Check sheet for the modelled part. Datum: model origin and axes. Units: mm. A direction names the side the tool comes from. Round coordinates to 2 decimals unless told otherwise and drop trailing zeros. Loops run counter-clockwise (first coordinate to the right, second up) from the corner with the lowest first, then second, coordinate; pieces in that order, holes last. Notation, with made-up numbers: (44, 53.5) - (76, 53.5) arc R22 ccw to (76, 81.5) - close; hole circle Ø5 at (13, 69). An arc over 180 degrees is marked (long way). Answer in a Markdown table with one row per item. Add a question column.
(1) Mould release check, pull along Z, two halves, no side actions. Record for faces 1 (the flat face through (2, -129, 637.838)), 2 (the flat face through (2, -905, 0)), 3 (the cylindrical face through (0.71, 158.39, -294.93)), 4 (the flat face through (127, -745, 362)): +Z half, -Z half, draft (parallel to the pull), parting line (faces both ways), or undercut.
(2) Cross-section at A-A on z = -132. Enter the section's corners in (x, y).
(3) Gauge pin test, flat ends, axial feed: pin 1 (10 mm diameter, centred on y = -849, z = 333.5, fed in from -X); pin 2 (1 mm diameter, centred on x = 78.5, z = 631.5, fed in from -Y); pin 3 (19 mm diameter, centred on x = -86, y = -46, fed in from -Z). Record the tip position at first contact, or that the pin passes through.
(4) Thickness scan on line 1 along X through (y, z) = (-1523, -123.5); line 2 along Y through (x, z) = (86.5, 217); line 3 along Z through (x, y) = (-113.5, -1066.5). Record the ranges inside material, lowest first.
(5) Cross-section at D-D on x = 187.5. Enter the section's corners in (y, z), then the cut area to 3 significant figures.
(6) Cross-section at C-C on z = 72.5. Enter the section's corners in (x, y), then the cut area to 3 significant figures.
(7) Access from +Z, -Z, +X, -X, +Y, -Y to the whole of each face (thin tool, end or side, straight path). Record for faces 5 (the flat face through (1.78, -223.03, 330.75)), 6 (the flat face through (-12.7, -380, 90)), 7 (the flat face through (12.7, -380, 90)), 8 (the flat face through (-400, -511, 923)), 9 (the flat face through (1.8, -167.7, 567.3)).
(8) Cross-section at B-B on y = -1586. Enter the section's corners in (x, z).
from build123d import *

# Parameters (mm, degrees)
F0_R      = 266.7
F1_DEPTH  = 38.1
F0_R_2    = 228.6
F2_DEPTH  = 50.8
F3_W      = 1447.8
F3_H      = 177.8
F4_DEPTH  = 12.7
F6_DEPTH  = 127
F7_R      = 325.686391
F7_R_2    = 334.768368
F8_DEPTH  = 50.8
F9_R      = 70.609631
F10_DEPTH = 400


with BuildPart() as f1:
    # F0 (on Right) → F1 (new body, symmetric)
    with BuildSketch(Plane.YZ):
        Circle(F0_R)
    extrude(amount=F1_DEPTH, both=True)



with BuildPart() as f2:
    # F0 (on Right) → F2 (new body, symmetric)
    with BuildSketch(Plane.YZ):
        with Locations((-1447.8, 0)):
            Circle(F0_R_2)
    extrude(amount=F2_DEPTH, both=True)


with BuildPart() as f1_1:
    add(f1.part)

    add(f2.part)  # F4 merges F2
    # F3 (on Right) → F4 (join, symmetric)
    with BuildSketch(Plane.YZ):
        with Locations((-723.9, 88.9)):
            Rectangle(F3_W, F3_H)
    extrude(amount=F4_DEPTH, both=True)

    # F5 (on Right) → F6 (join, symmetric)
    with BuildSketch(Plane.YZ):
        Polygon((-848.037601, 592.394769), (-1672.220111, 654.363334), (-1021.323022, 211.851792), (-1459.461212, 0), (-1219.849229, 0), (-438.957124, 0), (-438.957124, 478.463715), (-321.835073, 535.095428), (-63.101806, 0), (0, 0), (-263.467014, 544.885457), (-69.298647, 590.329111), (52.57291, 544.885457), (209.560111, 515.966773), (0, 637.838423), (-261.401385, 637.838423), (-279.991955, 753.513157), (-447.307229, 922.894001), (-509.275854, 922.894001), (-509.275854, 656.428993), (-558.850706, 685.347676), align=None)
    extrude(amount=F6_DEPTH, both=True)

    # F7 (on Right) → F8 (join, symmetric)
    with BuildSketch(Plane.YZ):
        with Locations((-1438.704967, 0)):
            Circle(F7_R)
        Circle(F7_R_2)
    extrude(amount=F8_DEPTH, both=True)

    # F9 (on Right) → F10 (join, symmetric)
    with BuildSketch(Plane.YZ):
        with Locations((-509.713531, 921.78303)):
            Circle(F9_R)
    extrude(amount=F10_DEPTH, both=True)


solid = f1_1.part
Answers:
| question | item | result |
|---|---|---|
| 1 | face 1 | +Z half |
| 1 | face 2 | -Z half |
| 1 | face 3 | undercut |
| 1 | face 4 | draft |
| 2 | outline | (-50.8, -1736.44) - (50.8, -1736.44) - (50.8, -1140.97) - (-50.8, -1140.97) - close; (-50.8, -307.65) - (50.8, -307.65) - (50.8, 307.65) - (-50.8, 307.65) - close |
| 3 | pin 1 | stops at x = -127 |
| 3 | pin 2 | stops at y = -1639.33 |
| 3 | pin 3 | stops at z = 0 |
| 4 | line 1 | x = -50.8 to 50.8 |
| 4 | line 2 | y = -1028.9 to -438.96, -168.03 to -104.93 |
| 4 | line 3 | z = 0 to 190.01, 242.57 to 608.82 |
| 5 | outline | circle Ø141.22 at (-509.71, 921.78) |
| 5 | area | 15,700 mm^2 |
| 6 | outline | (-127, -1309.52) - (-50.8, -1309.52) - (-50.8, -1756.22) - (50.8, -1756.22) - (50.8, -1309.52) - (127, -1309.52) - (127, -438.96) - (12.7, -438.96) - (12.7, -326.82) - (50.8, -326.82) - (50.8, -98.16) - (127, -98.16) - (127, -35.06) - (50.8, -35.06) - (50.8, 326.82) - (-50.8, 326.82) - (-50.8, -35.06) - (-127, -35.06) - (-127, -98.16) - (-50.8, -98.16) - (-50.8, -326.82) - (-12.7, -326.82) - (-12.7, -438.96) - (-127, -438.96) - close |
| 6 | area | 345,000 mm^2 |
| 7 | face 5 | none |
| 7 | face 6 | -X |
| 7 | face 7 | +X |
| 7 | face 8 | +Z, -Z, -X, +Y, -Y |
| 7 | face 9 | +X, -X |
| 8 | outline | (-127, 595.75) - (127, 595.75) - (127, 647.88) - (-127, 647.88) - close; (-50.8, -290.48) - (50.8, -290.48) - (50.8, 290.48) - (-50.8, 290.48) - close |
